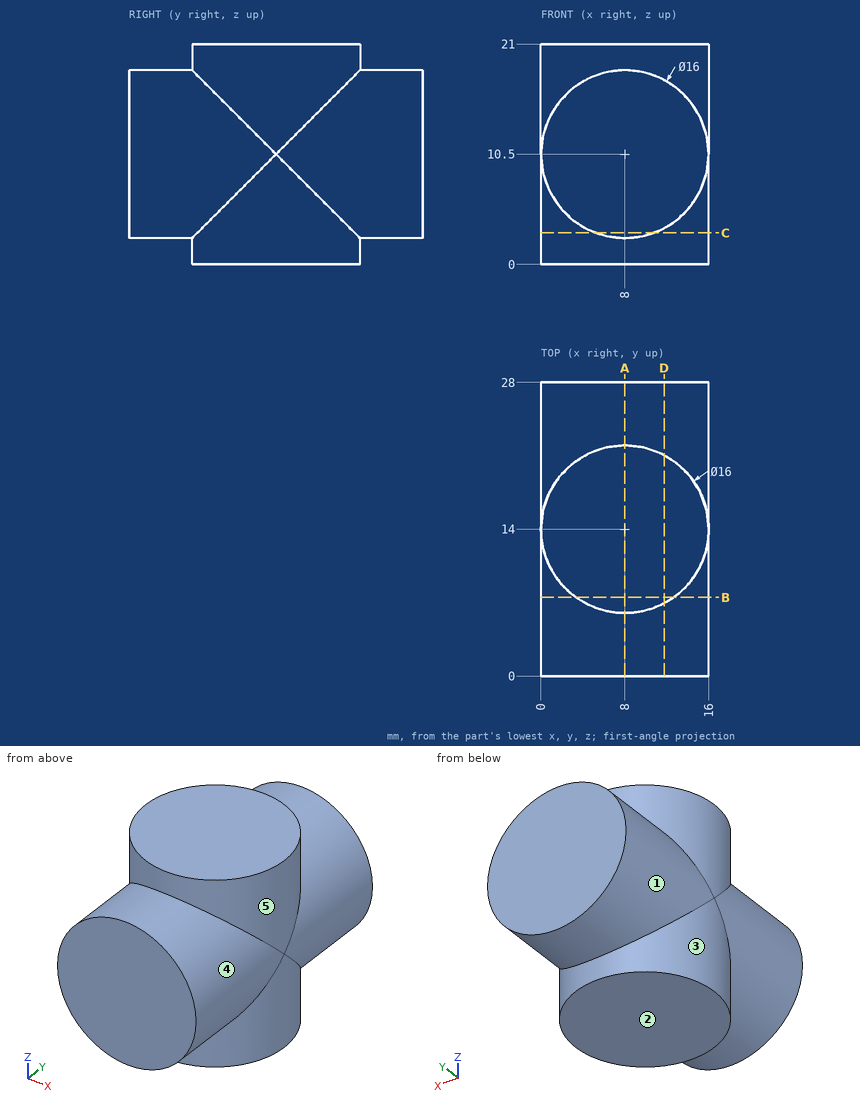
The figure shows three views and two pictorial views of one solid part (mm, origin at its lowest corner). Answer the questions. A direction names the side the tool comes from. Coordinates: 2 decimals unless noted, no trailing zeros. Loops run counter-clockwise (first coordinate to the right, second up) from the corner with the lowest first, then second, coordinate; pieces in that order, holes last. Notation, with made-up numbers: (-6.75, 63.5) - (20.25, 63.5) arc R17 cw to (20.25, 78.5) - close; hole circle Ø1 at (25.25, 20.5). An arc over 180 degrees is marked (long way). Answer in a Markdown table with one row per item.
Q1. Find section B-B on y = 7.5. Write down the section's boundary in (x, z).
Here are the results:
| item | result |
|---|---|
| outline | (3.34, 0) - (12.66, 0) - (12.66, 4) arc R8 ccw to (12.66, 17) - (12.66, 21) - (3.34, 21) - (3.34, 17) arc R8 ccw to (3.34, 4) - close |
Q2. Find section C-C on z = 3. Write down the section's boundary in (x, y), plus the area to 3 significant figures.
Here are the results:
| item | result |
|---|---|
| outline | (5.22, 0) - (10.78, 0) - (10.78, 6.5) arc R8 ccw to (10.78, 21.5) - (10.78, 28) - (5.22, 28) - (5.22, 21.5) arc R8 ccw to (5.22, 6.5) - close |
| area | 270 mm^2 |
Q3. For the marked faces 1, 2, 3, 4 and 5, determine the directions among +Z, -Z, +X, -X, +Y, -Y from which every point of the face is accessible in a straight line to the end or side of a thin tool.
Here are the results:
| item | result |
|---|---|
| face 1 | +Y |
| face 2 | -Z, +X, -X, +Y, -Y |
| face 3 | -Z |
| face 4 | -Y |
| face 5 | +Z |
Q4. Find section D-D on x = 11.75. Write down the section's boundary in (y, z), plus the area to 3 significant figures.
Here are the results:
| item | result |
|---|---|
| outline | (0, 3.43) - (6.93, 3.43) - (6.93, 0) - (21.07, 0) - (21.07, 3.43) - (28, 3.43) - (28, 17.57) - (21.07, 17.57) - (21.07, 21) - (6.93, 21) - (6.93, 17.57) - (0, 17.57) - close |
| area | 493 mm^2 |
Q5. Find section A-A on x = 8. Write down the section's boundary in (y, z), plus the area to 3 significant figures.
Here are the results:
| item | result |
|---|---|
| outline | (0, 2.5) - (6, 2.5) - (6, 0) - (22, 0) - (22, 2.5) - (28, 2.5) - (28, 18.5) - (22, 18.5) - (22, 21) - (6, 21) - (6, 18.5) - (0, 18.5) - close |
| area | 528 mm^2 |
Q6. Straight lines are drawn through the part: line 1 along Z through (x, y) = (8.25, 3); line 2 along X through (y, z) = (17.5, 2.5); line 3 along X through (y, z) = (8.25, 6). For each, find the intervals that lie inside material, in ascending order. Write a range as [from, to].
Here are the results:
| item | result |
|---|---|
| line 1 | z = [2.5, 18.5] |
| line 2 | x = [0.81, 15.19] |
| line 3 | x = [1.39, 14.61] |
Q7. Given P1, Ø1, axis at y = 9, z = 4.5, coming from the -X side; P2, Ø12, axis at y = 4.5, z = 18.5, coming from the -X side, each flat-ended and moving along its own axis, determine where each tip first touches the part or whether it passes through.
Here are the results:
| item | result |
|---|---|
| P1 | stops at x = 1.39 |
| P2 | stops at x = 0.25 |
